from build123d import *

# Parameters (mm, degrees)
F1_DEPTH  = 42
F2_W      = 75.478619273
F2_H      = 41.9138409197
F4_W      = 75.478619273
F4_H      = 41.9138409197
F5_DEPTH  = 3
F6_W      = 28
F6_H      = 12
F8_DEPTH  = 80
F11_W     = 100
F11_H     = 72.9077620213
F12_DEPTH = 7
F13_W     = 100
F13_H     = 72.9077620213
F13_W_2   = 94
F13_H_2   = 66.9077620213
F14_DEPTH = 2
F15_W     = 2
F15_H     = 0.5
F16_DEPTH = 0.5


# Not quite as in the source:
# - ends of sketch curves that miss each other by under 0.0002 mm in the source are joined
# - the dataset's text gives a spline's control points without its knots; the knots are read off the source's solid


with BuildPart() as f1:
    # F0 (on Top) → F1 (new body)
    with BuildSketch(Plane.XY):
        with BuildLine():
            Line((40.6705020705, 0), (45, 0))
            add(Edge.make_bspline(
                [(45, 0), (37.6566936716, 18.7177697445), (0.7563031661, 39.2432392178), (-39.1693000037, 19.753647335), (-45, 0)],
                knots=[0, 0, 0, 0, 0.5, 1, 1, 1, 1], degree=3))
            Line((-45, 0), (-40.8081785045, 0))
            add(Edge.make_bspline(
                [(40.6705020705, 0), (39.0654786869, 3.6685119371), (34.6366166878, 10.6499395063), (25.1941828283, 18.6625093529), (13.2155095249, 23.898149118), (2.1979882903, 25.5001155824), (-6.7612672319, 25.0396744323), (-15.5822493226, 23.419843787), (-23.8190972997, 20.0776830737), (-30.7940742115, 15.0930436532), (-35.2531784066, 10.5526098036), (-38.6097824931, 5.5150177421), (-40.2124471126, 1.7897260912), (-40.8081785045, 0)],
                knots=[0.0144696894, 0.0144696894, 0.0144696894, 0.0144696894, 0.125, 0.25, 0.375, 0.5, 0.5625, 0.625, 0.75, 0.8125, 0.875, 0.9375, 0.989221235, 0.989221235, 0.989221235, 0.989221235], degree=3))
        make_face()
    extrude(amount=F1_DEPTH)

    # F2 (on Front) → F3 (join, up to the next surface of F1)
    with BuildSketch(Plane.XZ):
        with Locations((-0.0689039235, 20.9569204599)):
            Rectangle(F2_W, F2_H)
    extrude(until=Until.NEXT, dir=(0, 1, 0))

    # F4 (on face) → F5 (join)
    with BuildSketch(Plane.XZ):
        with Locations((-0.0689039235, 20.9569204599)):
            Rectangle(F4_W, F4_H)
    extrude(amount=F5_DEPTH)

    # F6 (on Front) → F8 (join)
    with BuildSketch(Plane.XZ):
        with Locations((0, -6)):
            Rectangle(F6_W, F6_H)
    extrude(amount=-F8_DEPTH)

    # F11 (on face) → F12 (join)
    with BuildSketch(Plane(origin=(0, 11.8870032706, 28.3832509576), x_dir=(1, 0, 0), z_dir=(0, 0.3862941051, 0.9223756634))):
        with Locations((0, 77.4465687573)):
            Rectangle(F11_W, F11_H)
    extrude(amount=F12_DEPTH)

    # F13 (on face) → F14 (join)
    with BuildSketch(Plane(origin=(0, 14.591062006, 34.8398806013), x_dir=(1, 0, 0), z_dir=(0, 0.3862941051, 0.9223756634))):
        with Locations((0, 77.4465687573)):
            Rectangle(F13_W, F13_H)
        with Locations((0, 77.4465687573)):
            Rectangle(F13_W_2, F13_H_2, mode=Mode.SUBTRACT)
    extrude(amount=F14_DEPTH)

    # F15 (on face) → F16 (join)
    with BuildSketch(Plane(origin=(0, 15.3636502161, 36.684631928), x_dir=(1, 0, 0), z_dir=(0, 0.3862941051, 0.9223756634))):
        with Locations((33.4735295493, 42.3066589715)):
            Rectangle(F15_W, F15_H)
        with Locations((35.9735295493, 42.3066589715)):
            Rectangle(F15_W, F15_H)
        with Locations((38.4735295493, 42.3066589715)):
            Rectangle(F15_W, F15_H)
        with Locations((40.9735295493, 42.3066589715)):
            Rectangle(F15_W, F15_H)
        with Locations((30.9735295493, 42.3066589715)):
            Rectangle(F15_W, F15_H)
    extrude(amount=F16_DEPTH)


solid = f1.part
Design review of the part built by this model. Coordinates are the model's own, in mm. A direction names the side the tool comes from. Coordinates: 2 decimals unless noted, no trailing zeros. Loops run counter-clockwise (first coordinate to the right, second up) from the corner with the lowest first, then second, coordinate; pieces in that order, holes last. Notation, with made-up numbers: (51, 51) -> (63, 51) arc R11 cw to (63, 71) -> close; hole circle Ø10 at (17.5, 56). An arc over 180 degrees is marked (long way). Use a Markdown table: item, result. Add a question column.
Item 1: We need section C-C, the plane y = 108.5. Write out the cut boundary in (x, z), and give its area (3 significant figures).
Item 2: Wall thickness on L1, parallel to Z at x = -9.5, y = 76.5; L2, parallel to Z at x = 5, y = 11.5; L3, parallel to Y at x = -8.5, z = 5: over which ranges is each line inside the solid? List them lowest first. Write a range as from..to.
Item 3: We need section B-B, the plane z = -4. Write out the cut boundary in (x, y).
Item 4: We need section D-D, the plane y = 40.5. Write out the cut boundary in (x, z).
Item 5: Machinability: for faces 1 (the flat face through (-14, 39, -6)), 2 (the flat face through (-0.7, 51.41, 16.64)), 3 (the flat face through (14, 39, -6)), 4 (the flat face through (43, 0, 21)), 5 (the flat face through (0, 0, -6)), which of the approach directions +Z, -Z, +X, -X, +Y, -Y give a long, thin tool a straight path to every point of the face, cutting with its end or side? Answer none if there is none.
Item 6: We need section A-A, the plane y = 60. Write out the cut boundary in (x, z).
Item 7: The part is to be moulded in two halves that separate along Z. For faces 6 (the flat face through (-1, -3, 21)), 7 (the flat face through (0, 53, 0)), 8 (the flat face through (0, 39, -12)), say which applies: +Z half, -Z half, draft (parallel to the pull), parting line (faces both ways), or undercut.
Item 8: Clearance check with flat-ended pins moving along their axes: P1, Ø1.5, axis at y = 13, z = 34.5, coming from the +X side; P2, Ø5, axis at x = 42, z = 20, coming from the -Y side; P3, Ø12, axis at x = -30, y = 94, coming from the -Z side; P4, Ø0.5, axis at y = 54.5, z = 20.5, coming from the -X side. State where each tip first meets the part, or that it passes through.
Numbers:
| question | item | result |
|---|---|---|
| 1 | outline | (-50, -12.08) -> (50, -12.08) -> (50, -2.32) -> (47, -2.32) -> (47, -4.49) -> (-47, -4.49) -> (-47, -2.32) -> (-50, -2.32) -> close |
| 1 | area | 772 mm^2 |
| 2 | L1 | z = -12..0, 1.32..8.91 |
| 2 | L2 | z = -12..41.91 |
| 2 | L3 | y = -3..28.7, 67.72..85.84 |
| 3 | outline | (-50, 89.21) -> (50, 89.21) -> (50, 112.51) -> (47, 112.51) -> (47, 107.33) -> (-47, 107.33) -> (-47, 112.51) -> (-50, 112.51) -> close; (-14, 0) -> (14, 0) -> (14, 80) -> (-14, 80) -> close |
| 4 | outline | (-14, -12) -> (14, -12) -> (14, 0) -> (-14, 0) -> close |
| 5 | face 1 | -Z, -X, -Y |
| 5 | face 2 | +Z, +X, -X |
| 5 | face 3 | -Z, +X, -Y |
| 5 | face 4 | +Z, -Z, +X, -Y |
| 5 | face 5 | -Z, +X, -X, -Y |
| 6 | outline | (-50, 8.23) -> (50, 8.23) -> (50, 17.99) -> (47, 17.99) -> (47, 15.82) -> (-47, 15.82) -> (-47, 17.99) -> (-50, 17.99) -> close; (-14, -12) -> (14, -12) -> (14, 0) -> (-14, 0) -> close |
| 7 | face 6 | draft |
| 7 | face 7 | undercut |
| 7 | face 8 | -Z half |
| 8 | P1 | stops at x = 37.72 |
| 8 | P2 | stops at y = 0 |
| 8 | P3 | stops at z = -8.52 |
| 8 | P4 | stops at x = -50 |
